from build123d import *

# Parameters (mm, degrees)
F0_R     = 49.911
F1_DEPTH = 99.822
F4_DEPTH = 20.066


with BuildPart() as f1:
    # F0 (on Top) → F1 (new body)
    with BuildSketch(Plane.XY):
        Circle(F0_R)
    extrude(amount=F1_DEPTH)


with BuildPart() as f4:
    # F2 (on Top) → F4 (new body)
    with BuildSketch(Plane.XY):
        with BuildLine():
            Line((0, -49.6124997735), (0, 49.9553204259))
            ThreePointArc((0, 49.9553204259), (-49.6893893018, 0.1714103262), (0, -49.6124997735))
        make_face()
    extrude(amount=F4_DEPTH)


solid = f4.part
Check sheet for the modelled part. Datum: model origin and axes. Units: mm. Give positions to 0.01 mm unless a question says otherwise; leave off trailing zeros. Loops run counter-clockwise (first coordinate to the right, second up) from the corner with the lowest first, then second, coordinate; pieces in that order, holes last. Notation, with made-up numbers: M 6,67 L 13,67 A25 ccw 13,85 Z; hole C 22,63.25 d1. An arc over 180 degrees is marked long. Use a Markdown table: item, result. Add a question column.
Q1. Sectioned sample at B-B, the plane y = 21.5. Record the cut outline in (x, z), then the cut area to 3 significant figures.
Q2. Go/stop test with flat-tipped pins: pin 1 (4 mm diameter, centred on x = -39, z = 7, fed in from +Y); pin 2 (1 mm diameter, centred on y = 27.5, z = 5, fed in from -X); pin 3 (10 mm diameter, centred on x = -16, z = 15, fed in from -Y). Record where each tip stops, or that it passes through.
Q3. Sectioned sample at A-A, the plane z = 2.5. Record the cut outline in (x, y), then the cut area to 3 significant figures.
Q4. Scan lines: line 1 along X through (y, z) = (1, 7); line 2 along Y through (x, z) = (-23, 7.5); line 3 along Y through (x, z) = (-42.5, 14.5). Record each from-to range of solid material in increasing order. Write a range as [from, to].
Q5. Sectioned sample at C-C, the plane x = -12.5. Record the cut outline in (y, z), then the cut area to 3 significant figures.
Verdict:
| question | item | result |
|---|---|---|
| 1 | outline | M -44.89,0 L 0,0 L 0,20.07 L -44.89,20.07 Z |
| 1 | area | 901 mm^2 |
| 2 | pin 1 | y = 33.37 |
| 2 | pin 2 | x = -41.84 |
| 2 | pin 3 | y = -48.36 |
| 3 | outline | M 0,-49.61 L 0,49.96 A49.78 ccw Z |
| 3 | area | 3,880 mm^2 |
| 4 | line 1 | [-49.68, 0] |
| 4 | line 2 | [-43.93, 44.27] |
| 4 | line 3 | [-25.6, 25.94] |
| 5 | outline | M -47.99,0 L 48.34,0 L 48.34,20.07 L -47.99,20.07 Z |
| 5 | area | 1,930 mm^2 |
